Autodesk Inventor part; units mm, degrees
ref_plane "YZ Plane" through (0, 0, 0) normal (1, 0, 0) x (0, 1, 0)
ref_plane "XZ Plane" through (0, 0, 0) normal (0, 1, 0) x (-1, 0, 0)
ref_plane "XY Plane" through (0, 0, 0) normal (0, 0, 1) x (1, 0, 0)
sketch "Sketch6" plane through (0, 0, 0) normal (0, 0, 1) x (1, 0, 0)
  line L0 (-12.4, 5.9) -> (12.4, 5.9)
  line L1 (12.4, 5.9) -> (12.4, -5.9)
  line L2 (12.4, -5.9) -> (-12.4, -5.9)
  line L3 (-12.4, -5.9) -> (-12.4, 5.9)
  point P0 (0, 0)
  point P1 (-12.4, 0)
  point P2 (0, 5.9)
  dimension "d85" = 11.8
  dimension "d86" = 24.8
extrude "Extrusion3" add sketch "Sketch6" along normal blind 0.8
sketch "Sketch7" plane through (0, 0, 0.8) normal (0, 0, 1) x (1, 0, 0)
  point P0 (0, 0)
sketch "Sketch8" plane through (0, 0, 0.8) normal (0, 0, 1) x (1, 0, 0)
  line L0 (12.4, 5.9) -> (-12.4, 5.9)
  line L1 (-12.4, -5.9) -> (12.4, -5.9)
  line L2 (-12.4, 5.9) -> (-10.5276, 5.9)
  line L3 (-10.5276, -5.9) -> (-12.4, -5.9)
  line L4 (-12.4, -5.9) -> (-12.4, 5.9)
  line L5 (12.4, -5.9) -> (-10.5276, -5.9)
  line L6 (12.4163, 5.9) -> (10.7456, 5.9)
  line L7 (-12.4, 5.1) -> (11.6, 5.1)
  line L8 (11.6, 5.1) -> (11.6, -5.1)
  line L9 (11.6, -5.1) -> (-12.4, -5.1)
  line L10 (12.4, -5.9) -> (12.4, 5.9)
  point P0 (0, 0)
  dimension "d89" = 0.8
  dimension "d91" = 0.8
  dimension "d92" = 0.8
extrude "Extrusion4" add sketch "Sketch8" along normal blind 15 contours L10 L1 L4 L9 L8 L7 L0
sketch "Sketch9" plane through (-12.4, -5.9, 0) normal (-1, 0, 0) x (0, 0, 1)
  line L0 (0, 11.8) -> (15.8, 11.8)
  line L1 (0.8, 11) -> (15.8, 11)
  line L2 (15.8, 11.8) -> (15.8, 11)
  line L3 (15.8, 11) -> (0.8, 11)
  line L4 (0.8, 0.8) -> (15.8, 0.8)
  line L5 (0.8, 11) -> (0.8, 0.8)
  line L6 (0.8, 0.8) -> (15.8, 0.8)
  line L7 (0, 0) -> (15.8, 0)
  line L8 (15.8, 0.8) -> (15.8, 0)
  line L9 (15.8, 0) -> (0, 0)
  line L10 (0, 0) -> (0, 11.8)
  line L11 (0, 11.8) -> (15.8, 11.8)
  point P0 (0, 5.9)
  dimension "d95" = 0.8
extrude "Extrusion5" add sketch "Sketch9" along normal blind 10
properties part number "emax box"
Design review of the part built by this model. Coordinates are the model's own, in mm. A direction names the side the tool comes from. Coordinates: 2 decimals unless noted, no trailing zeros. Order: outer loops, then holes, each group sorted by start corner. A loop starts at its lowest first (then second) coordinate and runs counter-clockwise, first axis right, second up.
1) Clearance check with a flat-ended pin moving along its axis: pin 1 (4 mm diameter, centred on x = 0, y = 0, fed in from +Z). State where the tip first meets the part, or that it passes through.
2) Take a section at C-C, the plane z = 11.75. Give the boundary of the cut face in (x, y), and give its area (3 significant figures).
3) For faces 5 (the flat face through (-22.4, 5.3, 6.1)), 6 (the flat face through (-5, -5.1, 8)), list the 3-axis set-ups (+Z, -Z, +X, -X, +Y, -Y) from which the entire face can be reached by the end or side of a thin tool; tool diameter is ignored.
4) Wall thickness on line 1 along Y through (x, z) = (4, 6.5); line 2 along X through (y, z) = (2, 11.75); line 3 along Z through (x, y) = (-9.5, 4): over which ranges is each line inside the solid? List them lowest first.
5) Take a section at B-B, the plane y = 1.75. Give the boundary of the cut face in (x, z).
6) Mouldability with a two-part tool opening along Y and no side actions: class faces 1 (the flat face through (-5, 5.9, 8)), 2 (the flat face through (-5, 5.1, 8)), 3 (the flat face through (-2.3, 5.3, 15.8)), 4 (the flat face through (-5, 0, 0.8)) as +Y half, -Y half, draft (parallel to the pull), parting line (faces both ways), or undercut.
7) Take a section at A-A, the plane x = 1.5. Give the boundary of the cut face in (y, z).
Returned:
1. pin 1: stops at z = 0.8
2. outline: (-22.4, -5.9) - (12.4, -5.9) - (12.4, 5.9) - (-22.4, 5.9) - (-22.4, 5.1) - (11.6, 5.1) - (11.6, -5.1) - (-22.4, -5.1) - close
2. area: 63.8 mm2
3. face 5: +Z, -Z, -X, +Y, -Y
3. face 6: +Z, -X
4. line 1: y = -5.9 to -5.1, 5.1 to 5.9
4. line 2: x = 11.6 to 12.4
4. line 3: z = 0 to 0.8
5. outline: (-22.4, 0) - (12.4, 0) - (12.4, 15.8) - (11.6, 15.8) - (11.6, 0.8) - (-22.4, 0.8) - close
6. face 1: +Y half
6. face 2: undercut
6. face 3: draft
6. face 4: undercut
7. outline: (-5.9, 0) - (5.9, 0) - (5.9, 15.8) - (5.1, 15.8) - (5.1, 0.8) - (-5.1, 0.8) - (-5.1, 15.8) - (-5.9, 15.8) - close
